Input: dimensioned drawing with shaded views. Units: mm. Origin: part minimum x, y, z. A direction names the side the tool comes from. Round coordinates to 2 decimals unless told otherwise and drop trailing zeros. Loops run counter-clockwise (first coordinate to the right, second up) from the corner with the lowest first, then second, coordinate; pieces in that order, holes last. Notation, with made-up numbers: (4.25, 12.25) - (44.25, 12.25) arc R8 cw to (44.25, 16.25) - close; hole circle Ø4 at (48, -27.75). An arc over 180 degrees is marked (long way). Write each question's results on one line, items separated by ' | '.
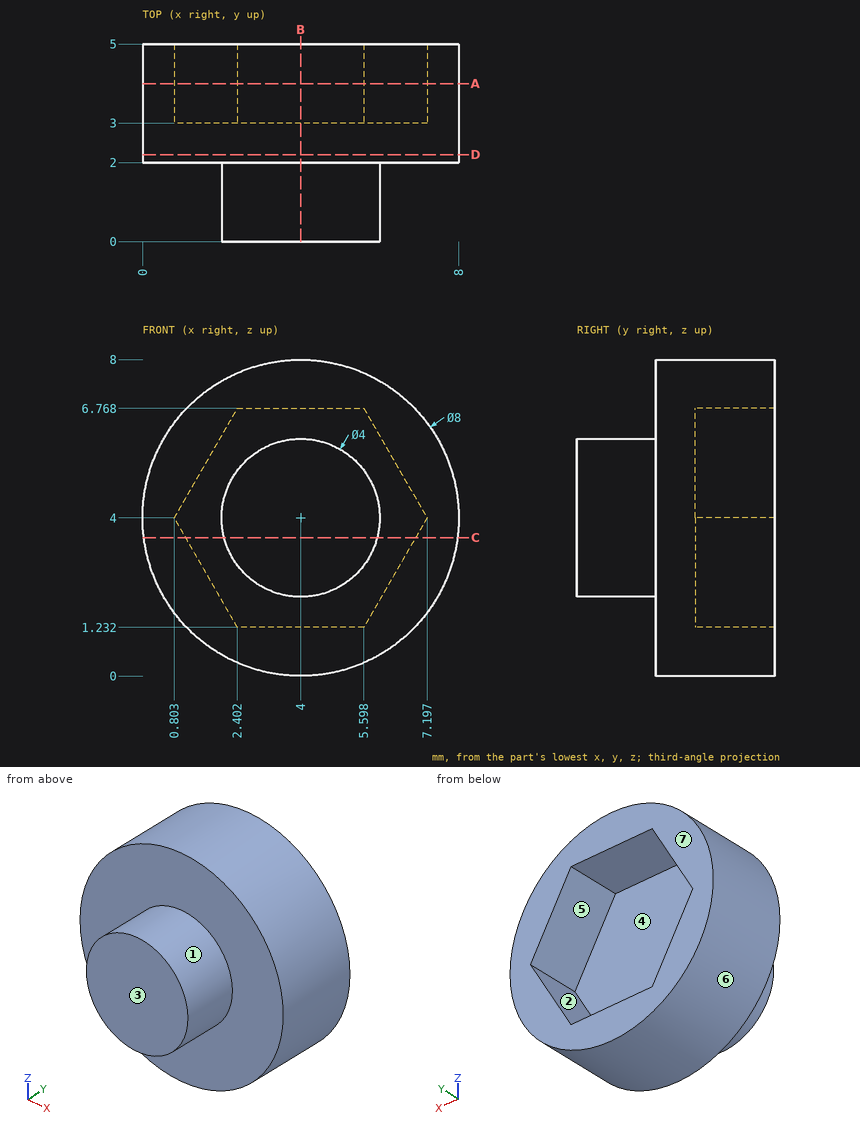
1. Line query: line 1 (Y direction, x = 3.5, z = 7.5); line 2 (Z direction, x = 3, y = 4.3); line 3 (Y direction, x = 4.5, z = 5). Output: solid intervals per line, ascending. Write a range as [from, to].
Answer:
line 1: [2, 5] | line 2: [0.13, 1.23], [6.77, 7.87] | line 3: [0, 3]
2. Section query A-A, the plane y = 4. Output: boundary loops of the cut face in (x, z).
Answer:
outline: circle Ø8 at (4, 4); hole (0.8, 4) - (2.4, 1.23) - (5.6, 1.23) - (7.2, 4) - (5.6, 6.77) - (2.4, 6.77) - close
3. Section query C-C, the plane z = 3.5. Output: boundary loops of the cut face in (x, y), plus the area to 3 significant figures.
Answer:
outline: (0.03, 2) - (2.06, 2) - (2.06, 0) - (5.94, 0) - (5.94, 2) - (7.97, 2) - (7.97, 5) - (6.91, 5) - (6.91, 3) - (1.09, 3) - (1.09, 5) - (0.03, 5) - close | area: 19.9 mm^2
4. Mould query, pull axis Z, two halves, no side actions, for the marked faces 4, 5, 6 and 7. Classes: pulls with the +Z half, pulls with the -Z half, needs draft (parallel to the pull), parting line crosses it, or undercut.
Answer:
face 4: undercut | face 5: undercut | face 6: parting line crosses it | face 7: needs draft
5. Contact query for flat-ended pins moving along their axis: pin 1 (2 mm diameter, centred on x = 3, y = 2, fed in from -Z); pin 2 (1.5 mm diameter, centred on x = 2, y = 1, fed in from +Z); pin 3 (1 mm diameter, centred on x = 3.5, z = 6, fed in from +Y); pin 4 (0.6 mm diameter, centred on x = 4.5, y = 4, fed in from +Z) (3 decimals). Output: stop coordinate, or through.
Answer:
pin 1: z = 0 | pin 2: z = 5.56 | pin 3: y = 3 | pin 4: z = 7.995
6. Section query B-B, the plane x = 4. Output: boundary loops of the cut face in (y, z).
Answer:
outline: (0, 2) - (2, 2) - (2, 0) - (5, 0) - (5, 1.23) - (3, 1.23) - (3, 6.77) - (5, 6.77) - (5, 8) - (2, 8) - (2, 6) - (0, 6) - close
7. Set-up query: the marked faces 1, 2 and 3. Return all of +Z, -Z, +X, -X, +Y, -Y with unobstructed straight access to the full face (end or side cutting, diameter ignored); none if empty.
Answer:
face 1: -Y | face 2: +Y | face 3: +Z, -Z, +X, -X, -Y
8. Section query D-D, the plane y = 2.2. Output: boundary loops of the cut face in (x, z).
Answer:
outline: circle Ø8 at (4, 4)
